Autodesk Inventor part; units mm, degrees
ref_plane "YZ Plane" through (0, 0, 0) normal (1, 0, 0) x (0, 1, 0)
ref_plane "XZ Plane" through (0, 0, 0) normal (0, 1, 0) x (-1, 0, 0)
ref_plane "XY Plane" through (0, 0, 0) normal (0, 0, 1) x (1, 0, 0)
sketch "Sketch1" plane through (0, 0, 0) normal (0, 1, 0) x (-1, 0, 0)
  line L0 (0, 0) -> (33, 0)
  line L1 (33, 0) -> (33, -70)
  line L2 (33, -70) -> (0, -70)
  line L3 (0, -70) -> (0, 0)
  dimension "d0" = 70
  dimension "d1" = 33
extrude "Extrusion1" add sketch "Sketch1" along normal blind 10
sketch "Sketch2" plane through (-33, 0, 0) normal (0, 0, 1) x (1, 0, 0)
  line L0 (14, 1.5) -> (29, 1.5)
  line L1 (14, 1.5) -> (14, 8.5)
  line L2 (14, 8.5) -> (29, 8.5)
  line L3 (29, 8.5) -> (29, 1.5)
  line L4 (14.5, 8) -> (28.5, 8)
  line L5 (28.5, 8) -> (28.5, 5)
  line L6 (28.5, 5) -> (14.5, 5)
  line L7 (14.5, 5) -> (14.5, 8)
  line L8 (33, 0) -> (33, 10)
  line L9 (33, 0) -> (0, 0)
  point P0 (21.5, 1.5)
  point P1 (30, -14)
  point P2 (21.5, 5)
  point P3 (30, -14)
  point P4 (30, -14)
  dimension "d4" = 15
  dimension "d5" = 7
  dimension "d6" = 14
  dimension "d7" = 3
  dimension "d8" = 0.5
  dimension "d9" = 0.5
  dimension "d22" = 4
  dimension "d23" = 1.5
extrude "Extrusion2" cut sketch "Sketch2" against normal blind 12
sketch "Sketch3" plane through (-33, 0, -70) normal (-1, 0, 0) x (0, 0, 1)
  line L0 (7, 1.5) -> (22, 1.5)
  line L1 (7, 1.5) -> (7, 8.5)
  line L2 (7, 8.5) -> (22, 8.5)
  line L3 (22, 8.5) -> (22, 1.5)
  line L4 (7.5, 8) -> (21.5, 8)
  line L5 (21.5, 8) -> (21.5, 5)
  line L6 (21.5, 5) -> (7.5, 5)
  line L7 (7.5, 5) -> (7.5, 8)
  line L8 (0, 0) -> (0, 10)
  line L9 (70, 0) -> (0, 0)
  line L10 (14.5, 8.5) -> (14.5, 1.5) construction
  line L11 (28, 1.5) -> (28, 8.5)
  line L12 (28.5, 5) -> (28.5, 8)
  line L13 (28.5, 8) -> (42.5, 8)
  line L14 (42.5, 8) -> (42.5, 5)
  line L15 (42.5, 5) -> (28.5, 5)
  line L16 (28, 1.5) -> (43, 1.5)
  line L17 (28, 8.5) -> (43, 8.5)
  line L18 (43, 8.5) -> (43, 1.5)
  line L19 (35.5, 8.5) -> (35.5, 1.5) construction
  line L20 (49, 1.5) -> (49, 8.5)
  line L21 (49.5, 5) -> (49.5, 8)
  line L22 (49.5, 8) -> (63.5, 8)
  line L23 (63.5, 8) -> (63.5, 5)
  line L24 (63.5, 5) -> (49.5, 5)
  line L25 (49, 1.5) -> (64, 1.5)
  line L26 (49, 8.5) -> (64, 8.5)
  line L27 (64, 8.5) -> (64, 1.5)
  line L28 (56.5, 8.5) -> (56.5, 1.5) construction
  point P0 (14.5, 5)
  point P1 (35.5, 5)
  point P2 (56.5, 5)
  dimension "d26" = 15
  dimension "d27" = 7
  dimension "d28" = 14
  dimension "d29" = 3
  dimension "d30" = 0.5
  dimension "d31" = 0.5
  dimension "d32" = 7
  dimension "d33" = 1.5
  dimension "d36" = 21
extrude "Extrusion3" cut sketch "Sketch3" against normal blind 12
sketch "Sketch4" plane through (0, 0, -70) normal (0, 0, -1) x (-1, 0, 0)
  circle A0 centre (16.5, 5) radius 1.5
  line L0 (33, 0) -> (0, 0)
  line L1 (0, 10) -> (33, 10)
  line L2 (0, 0) -> (0, 10)
  line L3 (33, 0) -> (33, 10)
  dimension "d43" = 3
  dimension "d44" = 10
  dimension "d45" = 33
  dimension "d46" = 5
  dimension "d47" = 16.5
extrude "Extrusion4" add sketch "Sketch4" along normal blind 10 contours A0
sketch "Sketch5" plane through (-16.5, 5, -80) normal (0, 0, -1) x (-1, 0, 0)
  circle A0 centre (0, 0) radius 1.5
  point P0 (-16.5, -5)
equation "\"d46\" = 0.5 * d44"
equation "\"d47\" = 0.5 * d45"
properties part number "usbHubSmall"
Source: CAD feature listing. Evaluate the final solid. Frame: model axes, mm. A direction names the side the tool comes from. Coordinates: 2 decimals unless noted, no trailing zeros. Order: outer loops, then holes, each group sorted by start corner. A loop starts at its lowest first (then second) coordinate and runs counter-clockwise, first axis right, second up. Notation, with made-up numbers: M 8,-16 L 12,-16 A22 ccw 12,5 Z; hole C -23,-18.75 d4. An arc over 180 degrees is marked long. Write each question's results on one line, items separated by ' | '. Start each with the question number.
Item 1: Cut plane C-C (x = -16.5). Return loops of the section in (y, z).
Item 2: Cut plane B-B (x = -23). Return loops of the section in (y, z).
Item 3: Set-up query: faces 4 (the face through (-12, 8, -6)), 5 (the face through (0, 5, -35)), 6 (the face through (-27, 8, -56)). Return all of +Z, -Z, +X, -X, +Y, -Y with unobstructed straight access to the full face (end or side cutting, diameter ignored); none if empty.
Item 4: Line query: probe 1 along Y at (x, z) = (-6.5, -10); probe 2 along Z at (x, y) = (-25, 3.5); probe 3 along X at (y, z) = (3, -8). Output: solid intervals per line, ascending.
Item 5: First-contact query: pin 1 Ø1.5 at (x, y) = (-26.5, 6.5) entering from -Z. Flat tip, straight axial feed; report the tip coordinate or a pass-through.
Item 6: Cut plane D-D (z = -54). Return loops of the section in (x, y).
Item 7: Draft query along Z for faces 1 (the face through (-11, 6, 0)), 2 (the face through (-15, 5, -75)), 3 (the face through (-27, 8.5, -56)). Return one class per face: pulls with the +Z half, pulls with the -Z half, needs draft (parallel to the pull), parting line crosses it, or undercut.
Item 8: Cut plane A-A (z = -8). Return loops of the section in (x, y).
Checked values:
1) outline: M 0,-70 L 3.5,-70 L 3.5,-80 L 6.5,-80 L 6.5,-70 L 10,-70 L 10,0 L 8.5,0 L 8.5,-12 L 8,-12 L 8,0 L 5,0 L 5,-12 L 1.5,-12 L 1.5,0 L 0,0 Z
2) outline: M 0,-70 L 10,-70 L 10,0 L 0,0 Z; M 5,-62.5 L 8,-62.5 L 8,-48.5 L 5,-48.5 Z; M 5,-41.5 L 8,-41.5 L 8,-27.5 L 5,-27.5 Z; M 5,-20.5 L 8,-20.5 L 8,-6.5 L 5,-6.5 Z; hole M 1.5,-63 L 8.5,-63 L 8.5,-48 L 1.5,-48 Z; hole M 1.5,-42 L 8.5,-42 L 8.5,-27 L 1.5,-27 Z; hole M 1.5,-21 L 8.5,-21 L 8.5,-6 L 1.5,-6 Z
3) face 4: +Z | face 5: +Z, -Z, +X, +Y, -Y | face 6: -X
4) probe 1: y = 0 to 1.5, 5 to 8, 8.5 to 10 | probe 2: z = -70 to -63, -48 to -42, -27 to -21, -6 to 0 | probe 3: x = -21 to -19, -4 to 0
5) pin 1: stops at z = -70
6) outline: M -33,0 L 0,0 L 0,10 L -33,10 L -33,8.5 L -21,8.5 L -21,8 L -33,8 L -33,5 L -21,5 L -21,1.5 L -33,1.5 Z
7) face 1: pulls with the +Z half | face 2: needs draft | face 3: undercut
8) outline: M -33,0 L 0,0 L 0,10 L -33,10 L -33,8.5 L -21,8.5 L -21,8 L -33,8 L -33,5 L -21,5 L -21,1.5 L -33,1.5 Z; M -18.5,5 L -4.5,5 L -4.5,8 L -18.5,8 Z; hole M -19,1.5 L -4,1.5 L -4,8.5 L -19,8.5 Z
